The model under review builds one solid part; all positions refer to its coordinate system, in mm. Face numbers are marked on the shaded views. A direction names the side the tool comes from. Round coordinates to 2 decimals unless told otherwise and drop trailing zeros. Loops run counter-clockwise (first coordinate to the right, second up) from the corner with the lowest first, then second, coordinate; pieces in that order, holes last. Notation, with made-up numbers: M -37.5,1.5 L -9.5,1.5 A15 cw -9.5,5.5 Z; hole C 15.25,30 d5. An arc over 180 degrees is marked long. Answer as a JSON object with one key per item and string values. Group by question number.
Item 1: Consider section C-C (x = 52). Give the boundary of the cut face in (y, z), and give its area (3 significant figures).
Item 2: The part is to be moulded in two halves that separate along X. For the marked faces 4, 5 and 6, say which applies: +X half, -X half, draft (parallel to the pull), parting line (faces both ways), or undercut.
Item 3: To check wall thickness, follow line 1 (X direction, y = -18.5, z = 83); line 2 (Z direction, x = 46.5, y = 0); line 3 (Z direction, x = 1.5, y = -15.5). State the ranges of each line that lie inside material, in increasing order.
Item 4: Consider section D-D (y = -27). Give the boundary of the cut face in (x, z), and give its area (3 significant figures).
Item 5: Insertion check: P1, Ø1, axis at y = -44.5, z = 12, coming from the -X side; P2, Ø18, axis at y = -13, z = 75, coming from the -X side; P3, Ø2, axis at y = -36, z = 54.5, coming from the -X side; P4, Ø8, axis at x = 29.5, y = 32.5, coming from the +Z side. Each pin has a flat end and moves straight along its axis. Give the tip position at first contact, or say it passes through.
Item 6: Consider section B-B (z = 19.5). Give the boundary of the cut face in (x, y), and give its area (3 significant figures).
Item 7: Tool access review of the marked faces 1, 2 and 3: name each direction out of +Z, -Z, +X, -X, +Y, -Y from which nothing blocks a thin tool from reaching the whole face with its end or side.
Item 8: Consider section A-A (z = 75). Give the boundary of the cut face in (x, y), and give its area (3 significant figures).
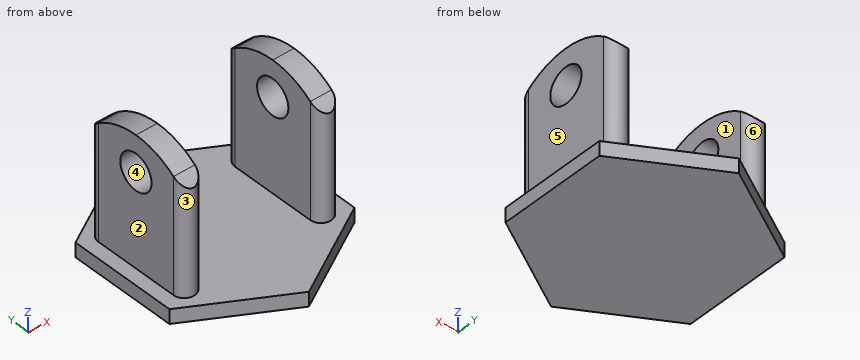
```python
from build123d import *

# Parameters (mm, degrees)
F1_DEPTH = 10
F3_DEPTH = 90
F4_R     = 12.5
F5_DEPTH = 120.4529052838


# Not quite as in the source:
# - a pattern or mirror of a feature is missing from the dataset's text; its kind, count and spacing are read off the source's solid


with BuildPart() as f1:
    # F0 (on Top) → F1 (new body)
    with BuildSketch(Plane.XY):
        Polygon((-64.9519052838, -37.5), (0, -75), (64.9519052838, -37.5), (64.9519052838, 37.5), (0, 75), (-64.9519052838, 37.5), align=None)
    extrude(amount=F1_DEPTH)

    # F2 (on face) → F3 (join)
    with BuildSketch(Plane.XY.offset(10)):
        with BuildLine():
            Line((-40.5, -30), (-40.5, 0))
            ThreePointArc((-40.5, 0), (-48, -7.5), (-55.5, 0))
            Line((-55.5, 0), (-55.5, -30))
            ThreePointArc((-55.5, -30), (-48, -37.5), (-40.5, -30))
        make_face()
        with BuildLine():
            ThreePointArc((-55.5, 0), (-48, -7.5), (-40.5, 0))
            ThreePointArc((-40.5, 0), (-48, 7.5), (-55.5, 0))
        make_face()
        with BuildLine():
            ThreePointArc((-55.5, 0), (-48, 7.5), (-40.5, 0))
            Line((-40.5, 0), (-40.5, 30))
            ThreePointArc((-40.5, 30), (-48, 37.5), (-55.5, 30))
            Line((-55.5, 30), (-55.5, 0))
        make_face()
    f3 = extrude(amount=F3_DEPTH)

    # F3_copies: F3 across plane
    add(f3.mirror(Plane(origin=(0, 0, 0), x_dir=(0, 0, 1), z_dir=(1, 0, 0))))

    # F4 (on face) → F5 (cut, through all)
    with BuildSketch(Plane(origin=(-55.5, 0, 0), x_dir=(0, -1, 0), z_dir=(-1, 0, 0))):
        with BuildLine():
            ThreePointArc((-38, 82.4961536185), (-34.2063872344, 86.4681103482), (-30, 90))
            Line((-30, 90), (-30, 100))
            Line((-30, 100), (-38, 100))
            Line((-38, 100), (-38, 82.4961536185))
        make_face()
        with BuildLine():
            ThreePointArc((-30, 90), (-15.8113883008, 97.4341649025), (0, 100))
            Line((0, 100), (-30, 100))
            Line((-30, 100), (-30, 90))
        make_face()
        with BuildLine():
            ThreePointArc((0, 100), (15.8113883008, 97.4341649025), (30, 90))
            Line((30, 90), (30, 100))
            Line((30, 100), (0, 100))
        make_face()
        with BuildLine():
            ThreePointArc((30, 90), (34.2063872344, 86.4681103482), (38, 82.4961536185))
            Line((38, 82.4961536185), (38, 100))
            Line((38, 100), (30, 100))
            Line((30, 100), (30, 90))
        make_face()
        with Locations((0, 75)):
            Circle(F4_R)
    extrude(amount=-F5_DEPTH, mode=Mode.SUBTRACT)


solid = f1.part
```
Geometry results:
{
 "1": {"outline": "M -44.98,0 L 44.98,0 L 44.98,10 L 36.34,10 L 36.34,84.34 A50 ccw -36.34,84.34 L -36.34,10 L -44.98,10 Z; hole C 0,75 d25", "area": "6,600 mm^2"},
 "2": {"face 4": "draft", "face 5": "+X half", "face 6": "undercut"},
 "3": {"line 1": "x = -55.5 to -40.5, 40.5 to 55.5", "line 2": "z = 0 to 62.5, 87.5 to 100", "line 3": "z = 0 to 10"},
 "4": {"outline": "M -64.95,0 L 64.95,0 L 64.95,10 L 55.5,10 L 55.5,92.08 L 40.5,92.08 L 40.5,10 L -40.5,10 L -40.5,92.08 L -55.5,92.08 L -55.5,10 L -64.95,10 Z", "area": "3,760 mm^2"},
 "5": {"P1": "passes through", "P2": "stops at x = -55.5", "P3": "stops at x = -53.59", "P4": "stops at z = 10"},
 "6": {"outline": "M -55.5,-30 A7.5 ccw -40.5,-30 L -40.5,30 A7.5 ccw -55.5,30 Z; M 40.5,-30 A7.5 ccw 55.5,-30 L 55.5,30 A7.5 ccw 40.5,30 Z", "area": "2,150 mm^2"},
 "7": {"face 1": "+Z, +Y, -Y", "face 2": "+Z, -X, +Y, -Y", "face 3": "+Z, -Y"},
 "8": {"outline": "M -55.5,-30 A7.5 ccw -40.5,-30 L -40.5,-12.5 L -55.5,-12.5 Z; M -55.5,12.5 L -40.5,12.5 L -40.5,30 A7.5 ccw -55.5,30 Z; M 40.5,-30 A7.5 ccw 55.5,-30 L 55.5,-12.5 L 40.5,-12.5 Z; M 40.5,12.5 L 55.5,12.5 L 55.5,30 A7.5 ccw 40.5,30 Z", "area": "1,400 mm^2"}
}
